Check sheet for the modelled part. Datum: model origin and axes. Units: mm. A direction names the side the tool comes from. Round coordinates to 2 decimals unless told otherwise and drop trailing zeros. Order: outer loops, then holes, each group sorted by start corner. A loop starts at its lowest first (then second) coordinate and runs counter-clockwise, first axis right, second up. Notation, with made-up numbers: (-30, 42) -> (5, 42) arc R24 ccw to (5, 55) -> close; hole circle Ø4 at (-36.75, 41). An arc over 180 degrees is marked (long way). Answer in a Markdown table with one row per item.
from build123d import *

# Parameters (mm, degrees)
F0_W     = 160
F0_H     = 15
F1_DEPTH = 10
F3_DEPTH = 5
F6_DEPTH = 3
F7_DEPTH = 10.001


with BuildPart() as f1:
    # F0 (on Front) → F1 (new body)
    with BuildSketch(Plane.XZ):
        Rectangle(F0_W, F0_H)
    extrude(amount=-F1_DEPTH)

    # F2 (on face) → F3 (cut)
    with BuildSketch(Plane(origin=(0, 10, 0), x_dir=(-1, 0, 0), z_dir=(0, 1, 0))):
        Polygon((58, 7.5), (-58, 7.5), (-49.339746, 2.5), (49.339746, 2.5), align=None)
        Polygon((-49.339746, -2.5), (-58, -7.5), (58, -7.5), (49.339746, -2.5), align=None)
    extrude(amount=-F3_DEPTH, mode=Mode.SUBTRACT)

    # F5 (on face) → F6 (cut)
    with BuildSketch(Plane(origin=(0, 10, 0), x_dir=(-1, 0, 0), z_dir=(0, 1, 0))):
        with BuildLine():
            ThreePointArc((-75, 3.5), (-78.5, 0), (-75, -3.5))
            Line((-75, -3.5), (-71, -3.5))
            ThreePointArc((-71, -3.5), (-67.5, 0), (-71, 3.5))
            Line((-71, 3.5), (-75, 3.5))
        make_face()
        with BuildLine():
            ThreePointArc((75, -3.5), (78.5, 0), (75, 3.5))
            Line((75, 3.5), (71, 3.5))
            ThreePointArc((71, 3.5), (67.5, 0), (71, -3.5))
            Line((71, -3.5), (75, -3.5))
        make_face()
    extrude(amount=-F6_DEPTH, mode=Mode.SUBTRACT)

    # F4 (on face) → F7 (cut, through all)
    with BuildSketch(Plane(origin=(0, 10, 0), x_dir=(-1, 0, 0), z_dir=(0, 1, 0))):
        with BuildLine():
            ThreePointArc((-75, 1.65), (-76.65, 0), (-75, -1.65))
            Line((-75, -1.65), (-71, -1.65))
            ThreePointArc((-71, -1.65), (-69.35, 0), (-71, 1.65))
            Line((-71, 1.65), (-75, 1.65))
        make_face()
        with BuildLine():
            ThreePointArc((75, -1.65), (76.65, 0), (75, 1.65))
            Line((75, 1.65), (71, 1.65))
            ThreePointArc((71, 1.65), (69.35, 0), (71, -1.65))
            Line((71, -1.65), (75, -1.65))
        make_face()
    extrude(amount=-F7_DEPTH, mode=Mode.SUBTRACT)


solid = f1.part
Item 1: Mould release check, pull along X, two halves, no side actions. Record for faces 6 (the flat face through (1, 8, 2.5)), 7 (the flat face through (-1, 0, 0)), 8 (the flat face through (-80, 5, 0)): pulls with the +X half, pulls with the -X half, needs draft (parallel to the pull), parting line crosses it, or undercut.
Result sheet:
| item | result |
|---|---|
| face 6 | undercut |
| face 7 | needs draft |
| face 8 | pulls with the -X half |
Item 2: Cross-section at B-B (y = 3.5). Record the boundary of the cut face in (x, z), and give its area (3 significant figures).
Result sheet:
| item | result |
|---|---|
| outline | (-80, -7.5) -> (80, -7.5) -> (80, 7.5) -> (-80, 7.5) -> close; hole (-75, -1.65) -> (-71, -1.65) arc R1.65 ccw to (-71, 1.65) -> (-75, 1.65) arc R1.65 ccw to start; hole (71, -1.65) -> (75, -1.65) arc R1.65 ccw to (75, 1.65) -> (71, 1.65) arc R1.65 ccw to start |
| area | 2,360 mm^2 |
Item 3: Cross-section at C-C (x = 3). Record the boundary of the cut face in (y, z), and give its area (3 significant figures).
Result sheet:
| item | result |
|---|---|
| outline | (0, -7.5) -> (5, -7.5) -> (5, -2.5) -> (10, -2.5) -> (10, 2.5) -> (5, 2.5) -> (5, 7.5) -> (0, 7.5) -> close |
| area | 100 mm^2 |
Item 4: Set-up check for faces 1 (the flat face through (-73, 9, -3.5)), 2 (the cylindrical face through (76.65, 3.55, 0.04)), 3 (the flat face through (-1, 10, 0)), 4 (the flat face through (-53.609, 7.535, 4.965)), 5 (the flat face through (53.609, 7.535, -4.965)): record each of +Z, -Z, +X, -X, +Y, -Y from which the full face is reachable in a straight line by a thin tool's end or side.
Result sheet:
| item | result |
|---|---|
| face 1 | +Y |
| face 2 | +Y, -Y |
| face 3 | +Z, -Z, +X, -X, +Y |
| face 4 | +Z, +Y |
| face 5 | -Z, +Y |
Item 5: Cross-section at D-D (z = 5.75). Record the boundary of the cut face in (x, y), and give its area (3 significant figures).
Result sheet:
| item | result |
|---|---|
| outline | (-80, 0) -> (80, 0) -> (80, 10) -> (54.97, 10) -> (54.97, 5) -> (-54.97, 5) -> (-54.97, 10) -> (-80, 10) -> close |
| area | 1,050 mm^2 |
Item 6: Depth check by flat-ended pin: P1, Ø1.5, axis at x = -11.5, z = 5.5, coming from the +Y side; P2, Ø2.5, axis at x = -8.5, y = 7, coming from the +Z side; P3, Ø5.5, axis at x = 74.5, z = 0, coming from the +Y side. Enter the tip coordinate at first touch or a pass-through.
Result sheet:
| item | result |
|---|---|
| P1 | stops at y = 5 |
| P2 | stops at z = 2.5 |
| P3 | stops at y = 7 |
Item 7: Cross-section at A-A (z = 0). Record the boundary of the cut face in (x, y), and give its area (3 significant figures).
Result sheet:
| item | result |
|---|---|
| outline | (-80, 0) -> (-76.65, 0) -> (-76.65, 7) -> (-78.5, 7) -> (-78.5, 10) -> (-80, 10) -> close; (-69.35, 0) -> (69.35, 0) -> (69.35, 7) -> (67.5, 7) -> (67.5, 10) -> (-67.5, 10) -> (-67.5, 7) -> (-69.35, 7) -> close; (76.65, 0) -> (80, 0) -> (80, 10) -> (78.5, 10) -> (78.5, 7) -> (76.65, 7) -> close |
| area | 1,430 mm^2 |
Item 8: Scan lines: line 1 (X direction, y = 1.75, z = -0.25); line 2 (Z direction, x = -35, y = 8.25); line 3 (X direction, y = 6.25, z = -4). Record each from-to range of solid material in increasing order. Write a range as [from, to].
Result sheet:
| item | result |
|---|---|
| line 1 | x = [-80, -76.63], [-69.37, 69.37], [76.63, 80] |
| line 2 | z = [-2.5, 2.5] |
| line 3 | x = [-80, -51.94], [51.94, 80] |
